Geometry check sheet. Reference: the model listing, model coordinates, mm. A direction names the side the tool comes from. Give positions to 0.01 mm unless a question says otherwise; leave off trailing zeros. Order: outer loops, then holes, each group sorted by start corner. A loop starts at its lowest first (then second) coordinate and runs counter-clockwise, first axis right, second up.
Autodesk Inventor part; units mm, degrees
ref_plane "YZ Plane" through (0, 0, 0) normal (1, 0, 0) x (0, 1, 0)
ref_plane "XZ Plane" through (0, 0, 0) normal (0, 1, 0) x (-1, 0, 0)
ref_plane "XY Plane" through (0, 0, 0) normal (0, 0, 1) x (1, 0, 0)
sketch "Skizze_Grundkörper" plane through (0, 0, 0) normal (0, 0, 1) x (1, 0, 0)
  line L0 (-63, 0) -> (63, 0)
  line L1 (0, -63) -> (0, 63)
  line L2 (45, -45) -> (-45, -45)
  line L3 (-45, -45) -> (-45, 45)
  line L4 (-45, 45) -> (45, 45)
  line L5 (45, 45) -> (45, -45)
  line L6 (45, -45) -> (-45, 45) construction
  line L7 (-45, -45) -> (45, 45) construction
  point P0 (0, 0)
  dimension "Breite" = 90
  dimension "Länge" = 90
extrude "Grundkörper" add sketch "Skizze_Grundkörper" along normal mid plane 10
sketch "Skizze_Senkbohrung" plane through (0, 0, 5) normal (0, 0, 1) x (1, 0, 0)
  line L0 (-63, 0) -> (63, 0)
  line L1 (0, -63) -> (0, 63)
  point P0 (0, 0)
  point P1 (-18.5, 0)
  point P2 (18.5, 0)
  dimension "Senkbohrung_Abstand" = 37
hole "Senkbohrung" at (-18.5, 0, 5) at (18.5, 0, 5) direction (0, 0, -1) diameter 4.5 end through all counterbore diameter 8 counterbore depth 4.4
sketch "Skizze_Gewindebohrung_M5" plane through (0, 0, 5) normal (0, 0, 1) x (1, 0, 0)
  line L0 (-63, 0) -> (63, 0)
  line L1 (0, -63) -> (0, 63)
  point P0 (0, 0)
  point P1 (-38, 0)
  point P2 (38, 0)
  dimension "Gewindeabstand" = 76
hole "Gewindebohrung_M5" at (-38, 0, 5) at (38, 0, 5) direction (0, 0, -1) diameter 4.134 end through all
properties part number "Grundplatte_2016_iLogic"
Item 1: Draft check along X on faces 3 (the flat face through (45, 1, 0)), 4 (the cylindrical face through (14.534, 0.521, 2.769)), 5 (the flat face through (1, -45, 0)), 6 (the flat face through (-45, -1, 0)). Enter one of: released by +X, released by -X, zero draft, split by the parting line, or undercut.
Reported:
face 3: released by +X
face 4: undercut
face 5: zero draft
face 6: released by -X
Item 2: Set-up check for faces 1 (the flat face through (-1, 45, 0)), 2 (the flat face through (-17, -2, 0.6)): record each of +Z, -Z, +X, -X, +Y, -Y from which the full face is reachable in a straight line by a thin tool's end or side.
Reported:
face 1: +Z, -Z, +X, -X, +Y
face 2: +Z
Item 3: Sectioned sample at C-C (x = 38). Enter the section's corners in (y, z).
Reported:
outline: (-45, -5) - (-2.07, -5) - (-2.07, 5) - (-45, 5) - close; (2.07, -5) - (45, -5) - (45, 5) - (2.07, 5) - close
Item 4: Scan lines: L1, parallel to X at y = 0, z = 2.75; L2, parallel to Y at x = 18.5, z = -2.4; L3, parallel to Y at x = 18.5, z = 1.65. Record each from-to range of solid material in increasing order.
Reported:
L1: x = -45 to -40.07, -35.93 to -22.5, -14.5 to 14.5, 22.5 to 35.93, 40.07 to 45
L2: y = -45 to -2.25, 2.25 to 45
L3: y = -45 to -4, 4 to 45
Item 5: Sectioned sample at B-B (y = 0). Enter the section's corners in (x, z).
Reported:
outline: (-45, -5) - (-40.07, -5) - (-40.07, 5) - (-45, 5) - close; (-35.93, -5) - (-20.75, -5) - (-20.75, 0.6) - (-22.5, 0.6) - (-22.5, 5) - (-35.93, 5) - close; (-16.25, -5) - (16.25, -5) - (16.25, 0.6) - (14.5, 0.6) - (14.5, 5) - (-14.5, 5) - (-14.5, 0.6) - (-16.25, 0.6) - close; (20.75, -5) - (35.93, -5) - (35.93, 5) - (22.5, 5) - (22.5, 0.6) - (20.75, 0.6) - close; (40.07, -5) - (45, -5) - (45, 5) - (40.07, 5) - close
Item 6: Gauge pin test, flat end, axial feed: pin 1 (6.5 mm diameter, centred on x = -18.5, y = 0, fed in from -Z). Record the tip position at first contact, or that the pin passes through.
Reported:
pin 1: stops at z = -5
Item 7: Sectioned sample at A-A (x = -18.5). Enter the section's corners in (y, z).
Reported:
outline: (-45, -5) - (-2.25, -5) - (-2.25, 0.6) - (-4, 0.6) - (-4, 5) - (-45, 5) - close; (2.25, -5) - (45, -5) - (45, 5) - (4, 5) - (4, 0.6) - (2.25, 0.6) - close
